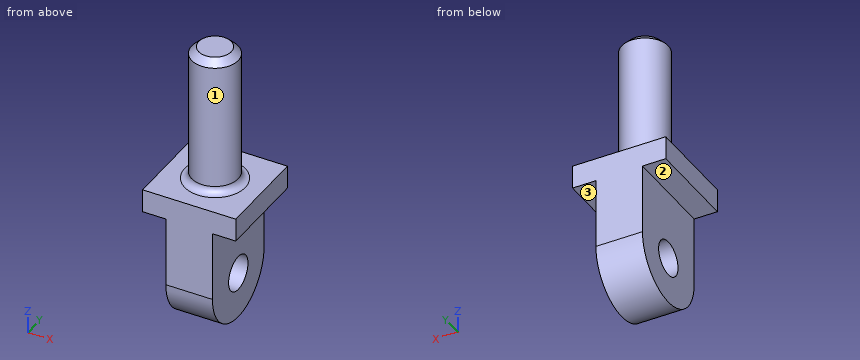
from build123d import *

# Parameters (mm, degrees)
SKETCH1_W         = 50.8
SKETCH1_H         = 50.8
SQUARE_BASE_DEPTH = 12.7
SKETCH2_R         = 12.7
LONG_PIN_DEPTH    = 76.2
SKETCH3_R         = 9.525
EYELET_DEPTH      = 12.7
FILLET1_R         = 3.81
CHAMFER1_SIZE     = 3.81


with BuildPart() as part:
    # Sketch1 → Square Base (new body)
    with BuildSketch(Plane.XY):
        Rectangle(SKETCH1_W, SKETCH1_H)
    extrude(amount=-SQUARE_BASE_DEPTH)

    # Sketch2 → Long Pin (add)
    with BuildSketch(Plane.XY):
        with Locations(Location((0, 0, 0), (0, 0, 180))):
            Circle(SKETCH2_R)
    extrude(amount=LONG_PIN_DEPTH)

    # Sketch3 → Eyelet (add, symmetric)
    with BuildSketch(Plane(origin=(0, 0, 0), x_dir=(0, 0, -1), z_dir=(1, 0, 0))):
        with BuildLine():
            Line((12.7, 25.4), (50.8, 25.4))
            ThreePointArc((50.8, 25.4), (76.2, 0), (50.8, -25.4))
            Line((50.8, -25.4), (12.7, -25.4))
            Line((12.7, -25.4), (12.7, 25.4))
        make_face()
        with Locations((50.8, 0)):
            Circle(SKETCH3_R, mode=Mode.SUBTRACT)
    extrude(amount=EYELET_DEPTH, both=True)

    # Fillet1
    fillet1_edges = [part.edges().sort_by_distance(p)[0] for p in [
        (12.7, 0, 0),
    ]]
    fillet(fillet1_edges, radius=FILLET1_R)

    # Chamfer1
    chamfer1_edges = [part.edges().sort_by_distance(p)[0] for p in [
        (12.7, 0, 76.2),
    ]]
    chamfer(chamfer1_edges, length=CHAMFER1_SIZE)


solid = part.part
Source: CAD feature listing. Evaluate the final solid. Frame: model axes, mm. Face numbers are marked on the shaded views. A direction names the side the tool comes from. Give positions to 0.01 mm unless a question says otherwise; leave off trailing zeros. Write each loop counter-clockwise with the first axis right and the second up, starting at its lowest first coordinate (ties: lowest second). Pieces come first, ordered by that corner, then holes. Notation, with made-up numbers: M -0.75,-28 L 28.25,-28 A17 cw 28.25,-2 Z; hole C 58.25,17 d1. An arc over 180 degrees is marked long. Return JSON: item names as keys, results as strings. Group by question number.
1) Cut plane C-C, the plane z = -16.5. Output: boundary loops of the cut face in (x, y), then the cut area to 3 significant figures.
2) First-contact query: pin 1 Ø6 at (y, z) = (12, -27.5) entering from +X; pin 2 Ø8 at (y, z) = (-15, -51) entering from -X; pin 3 Ø1.5 at (x, z) = (-7.5, 7.5) entering from -Y. Flat tips, straight axial feed; report the tip coordinate or a pass-through.
3) Cut plane A-A, the plane y = 0. Output: boundary loops of the cut face in (x, z) (3 decimals).
4) Cut plane B-B, the plane x = 0. Output: boundary loops of the cut face in (y, z) (3 decimals), then the cut area to 3 significant figures.
5) Set-up query: the marked faces 1, 2 and 3. Return all of +Z, -Z, +X, -X, +Y, -Y with unobstructed straight access to the full face (end or side cutting, diameter ignored); none if empty.
6) Cut plane D-D, the plane x = 20.5. Output: boundary loops of the cut face in (y, z), then the cut area to 3 significant figures.
7) Ray query, L1, parallel to Y at x = 0, z = -50; L2, parallel to Z at x = 20.5, y = -4; L3, parallel to X at y = 15, z = -59. Return the intervals inside material, ascending.
Data:
{
 "1": {"outline": "M -12.7,-25.4 L 12.7,-25.4 L 12.7,25.4 L -12.7,25.4 Z", "area": "1,290 mm²"},
 "2": {"pin 1": "stops at x = 12.7", "pin 2": "stops at x = -12.7", "pin 3": "stops at y = -10.76"},
 "3": {"outline": "M -25.4,-12.7 L -12.7,-12.7 L -12.7,-41.275 L 12.7,-41.275 L 12.7,-12.7 L 25.4,-12.7 L 25.4,0 L 16.51,0 A3.81 cw 12.7,3.81 L 12.7,72.39 L 8.89,76.2 L -8.89,76.2 L -12.7,72.39 L -12.7,3.81 A3.81 cw -16.51,0 L -25.4,0 Z; M -12.7,-76.2 L 12.7,-76.2 L 12.7,-60.325 L -12.7,-60.325 Z"},
 "4": {"outline": "M -25.4,-50.8 A25.4 ccw 25.4,-50.8 L 25.4,0 L 16.51,0 A3.81 cw 12.7,3.81 L 12.7,72.39 L 8.89,76.2 L -8.89,76.2 L -12.7,72.39 L -12.7,3.81 A3.81 cw -16.51,0 L -25.4,0 Z; hole C 0,-50.8 d19.05", "area": "5,240 mm²"},
 "5": {"face 1": "+Z", "face 2": "-Z, -X, +Y, -Y", "face 3": "-Z, +X, +Y, -Y"},
 "6": {"outline": "M -25.4,-12.7 L 25.4,-12.7 L 25.4,0 L -25.4,0 Z", "area": "645 mm²"},
 "7": {"L1": "y = -25.4 to -9.49, 9.49 to 25.4", "L2": "z = -12.7 to 0", "L3": "x = -12.7 to 12.7"}
}
